For this review, take the finished solid that the model builds, in its own axes (mm). Face numbers are marked on the shaded views. A direction names the side the tool comes from. Give positions to 0.01 mm unless a question says otherwise; leave off trailing zeros. Loops run counter-clockwise (first coordinate to the right, second up) from the corner with the lowest first, then second, coordinate; pieces in that order, holes last.
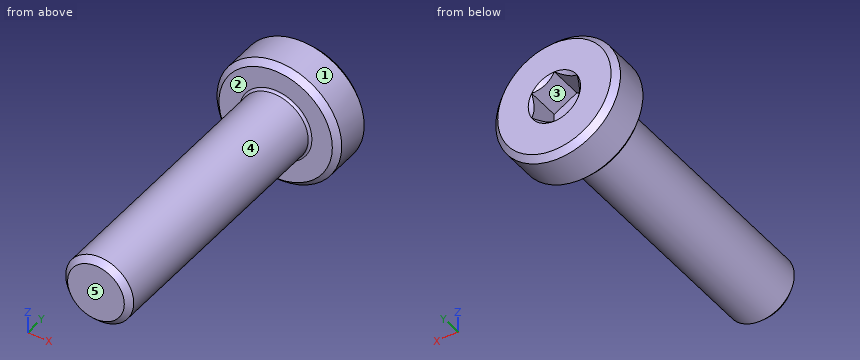
Autodesk Inventor part; units mm, degrees
ref_plane "YZ Plane" through (0, 0, 0) normal (1, 0, 0) x (0, 1, 0)
ref_plane "XZ Plane" through (0, 0, 0) normal (0, 1, 0) x (-1, 0, 0)
ref_plane "XY Plane" through (0, 0, 0) normal (0, 0, 1) x (1, 0, 0)
sketch "Sketch1" plane through (0, 0, 0) normal (0, 0, 1) x (1, 0, 0)
  line L0 (0, 7) -> (0, -7)
  line L1 (0, -7) -> (1.25, -7)
  line L2 (1.25, -7) -> (1.5, -6.75)
  line L3 (1.5, -6.75) -> (1.5, 4.9)
  line L4 (1.6, 5) -> (2.5, 5)
  line L5 (2.75, 5.25) -> (2.75, 6.75)
  line L6 (2.5, 7) -> (0, 7)
  arc A0 (1.6, 5) -> (1.5, 4.9) centre (1.6, 4.9) ccw
  line L7 (2.5, 7) -> (2.75, 6.75)
  line L8 (2.5, 5) -> (2.75, 5.25)
  point P0 (0, 0)
  point P1 (2.75, 5)
  point P2 (2.75, 7)
  point P3 (0, 0)
  dimension "d0" = 5.5
  dimension "d1" = 2
  dimension "d3" = 3
  dimension "d4" = 3.2
  dimension "d5" = 135
  dimension "d6" = 0.25
  dimension "d7" = 12
  dimension "d9" = 0.25
revolve "Revolution1" add sketch "Sketch1" angle 360 about axis through (0, 7, 0) along (0, -1, 0)
sketch "Sketch2" plane through (0, 7, 0) normal (0, 1, 0) x (1, 0, 0)
  line L0 (0, -1.1547) -> (-1, -0.5774)
  line L1 (-1, -0.5774) -> (-1, 0.5774)
  line L2 (-1, 0.5774) -> (0, 1.1547)
  line L3 (0, 1.1547) -> (1, 0.5774)
  line L4 (1, 0.5774) -> (1, -0.5774)
  line L5 (1, -0.5774) -> (0, -1.1547)
  point P0 (0, 0)
  point P1 (0, 0)
  dimension "d11" = 2
extrude "Extrusion1" cut sketch "Sketch2" against normal blind 1.5
thread "Thread1"
sketch "Sketch3" plane through (0, 0, 0) normal (1, 0, 0) x (0, 1, 0)
  line L0 (7, 1.1547) -> (6, 0.1547)
  line L1 (6, 0.1547) -> (7, 0.1547)
  line L2 (7, 0.1547) -> (7, 1.1547)
  line L3 (-1.4, 0) -> (8.4, 0)
  point P0 (0, 0)
  dimension "d18" = 1
revolve "Revolution2" cut sketch "Sketch3" angle 360 about axis through (0, -10, 0) along (0, 1, 0)
properties part number "Bolt_M3x0.35_12mm_SH" material "Stainless Steel"
Q1. For pin 1 Ø1.5 at (y, z) = (-3.5, 2) entering from -X; pin 2 Ø1.5 at (y, z) = (4, 0) entering from -X; pin 3 Ø1 at (x, z) = (2, -1) entering from -Y, all flat-tipped, find the tip position at first contact; note any pin that passes through.
Answers:
pin 1: stops at x = -0.83
pin 2: stops at x = -1.5
pin 3: stops at y = 5
Q2. For probe 1 along Y at (x, z) = (0.75, -0.35); probe 2 along Y at (x, z) = (0.4, -2.45); probe 3 along Z at (x, y) = (0.05, -2.5), list the stretches that pass through material, from the lowest coordinate up.
Answers:
probe 1: y = -7 to 5.5
probe 2: y = 5 to 7
probe 3: z = -1.5 to 1.5
Q3. Consider section A-A on z = 0. Give the boundary of the cut face in (x, y), plus the area to 3 significant figures.
Answers:
outline: (-2.75, 5.25) - (-2.5, 5) - (-1.6, 5) arc R0.1 cw to (-1.5, 4.9) - (-1.5, -6.75) - (-1.25, -7) - (1.25, -7) - (1.5, -6.75) - (1.5, 4.9) arc R0.1 cw to (1.6, 5) - (2.5, 5) - (2.75, 5.25) - (2.75, 6.75) - (2.5, 7) - (1.15, 7) - (1, 6.85) - (1, 5.5) - (-1, 5.5) - (-1, 6.85) - (-1.15, 7) - (-2.5, 7) - (-2.75, 6.75) - close
area: 43.8 mm2
Q4. Consider section B-B on y = 1.5. Give the boundary of the cut face in (x, z), plus the area to 3 significant figures.
Answers:
outline: circle Ø3 at (0, 0)
area: 7.07 mm2
Q5. Machinability: for the marked faces 1 and 2, which of the approach directions +Z, -Z, +X, -X, +Y, -Y give a long, thin tool a straight path to every point of the face, cutting with its end or side? Answer none if there is none.
Answers:
face 1: +Y, -Y
face 2: -Y
Q6. Mouldability with a two-part tool opening along X and no side actions: class the marked faces 3, 4 and 5 as +X half, -X half, draft (parallel to the pull), parting line (faces both ways), or undercut.
Answers:
face 3: undercut
face 4: parting line
face 5: draft
